Could you check a few things on this model? Use its own coordinates, in mm. Face numbers are marked on the shaded views. A direction names the side the tool comes from. Coordinates: 2 decimals unless noted, no trailing zeros. Order: outer loops, then holes, each group sorted by start corner. A loop starts at its lowest first (then second) coordinate and runs counter-clockwise, first axis right, second up. Notation, with made-up numbers: (20, 70.25) - (29, 70.25) arc R21 cw to (29, 107.25) - close; hole circle Ø10 at (41.5, 88). An arc over 180 degrees is marked (long way). Answer as a JSON object with one key per item and string values. Group by question number.
(1) Imagine slicing it at B-B, the plane z = 39. Write out the boundary of the cut face in (x, y), and give its area (3 significant figures).
(2) We'd pull the mould along X, two halves only. Please class the marked faces 3, 4, 5 and 6: pulls with the +X half, pulls with the -X half, needs draft (parallel to the pull), parting line crosses it, or undercut.
(3) Will these pins go through, and if not, where does the flat tip stop? P1, Ø1, axis at x = -30, y = -20.5, coming from the +Z side; P2, Ø0.6, axis at y = -58, z = 0.5, coming from the +X side; P3, Ø3, axis at y = 42.5, z = 10, coming from the +X side.
(4) Which directions (+Z, -Z, +X, -X, +Y, -Y) give clear straight access to the entire face, cutting with the end or side of a thin tool? Please do the marked faces 1 and 2.
(5) Please list where these lines run through material, in increasing order: probe 1 along X at (y, z) = (32, 39.5); probe 2 along X at (y, z) = (41, 45); probe 3 along Z at (x, y) = (-56, 97).
(6) Imagine slicing it at A-A, the plane x = -19.5. Write out the boundary of the cut face in (y, z).
(7) Imagine slicing it at C-C, the plane y = 83.5. Write out the boundary of the cut face in (x, z), and give its area (3 significant figures).
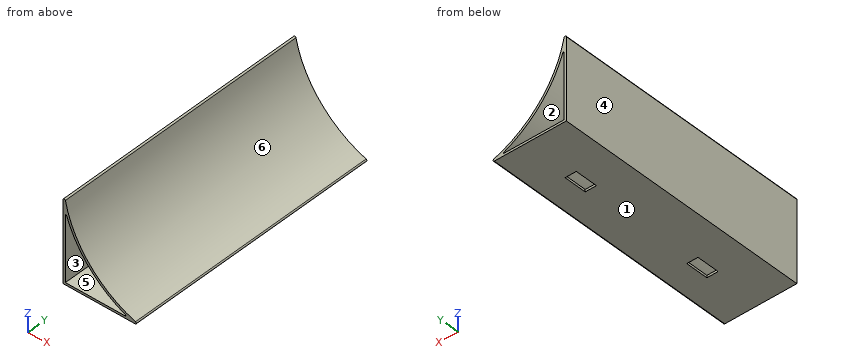
from build123d import *

# Parameters (mm, degrees)
BOSS_EXTRUDE1_DEPTH      = 113.5
BOSS_EXTRUDE1_DEPTH_BACK = 113.5
SKETCH3_W                = 9.8
SKETCH3_H                = 19.8
CUT_EXTRUDE1_DEPTH       = 5


with BuildPart() as part:
    # Sketch2 → Boss-Extrude1 (new, two sides: drawn at the far end of the back side and taken through both)
    with BuildSketch(Plane(origin=(0, 0, 0), x_dir=(-1, 0, 0), z_dir=(0, 1, 0)).offset(-BOSS_EXTRUDE1_DEPTH_BACK)):
        with BuildLine():
            Line((6.944925281, 0), (70, 0))
            Line((70, 0), (70, 70.727517767))
            ThreePointArc((70, 70.727517767), (69.10322059, 71.722176256), (68.02130898, 70.932856238))
            ThreePointArc((68.02130898, 70.932856238), (46.50806151, 28.267371652), (6.627399441, 1.948249619))
            ThreePointArc((6.627399441, 1.948249619), (5.957947667, 0.839142329), (6.944925281, 0))
        make_face()
        with BuildLine():
            Line((68, 58.856286255), (68, 2))
            Line((68, 2), (15.588847456, 2))
            ThreePointArc((15.588847456, 2), (15.099520976, 2.397240103), (15.387714901, 2.957761614))
            ThreePointArc((15.387714901, 2.957761614), (47.071395865, 25.58711402), (67.027291068, 59.019216502))
            ThreePointArc((67.027291068, 59.019216502), (67.582600042, 59.349416291), (68, 58.856286255))
        make_face(mode=Mode.SUBTRACT)
    extrude(amount=BOSS_EXTRUDE1_DEPTH + BOSS_EXTRUDE1_DEPTH_BACK)

    # Sketch3 → Cut-Extrude1 (cut)
    with BuildSketch(Plane(origin=(0, 0, 0), x_dir=(1, 0, 0), z_dir=(0, 0, -1))):
        with Locations((-35, -59.9)):
            Rectangle(SKETCH3_W, SKETCH3_H)
        with Locations((-35, 59.9)):
            Rectangle(SKETCH3_W, SKETCH3_H)
    extrude(amount=-CUT_EXTRUDE1_DEPTH, mode=Mode.SUBTRACT)


solid = part.part
Result set:
{
 "1": {"outline": "(-70, -113.5) - (-68, -113.5) - (-68, 113.5) - (-70, 113.5) - close; (-57.38, -113.5) - (-54.74, -113.5) - (-54.74, 113.5) - (-57.38, 113.5) - close", "area": "1,050 mm^2"},
 "2": {"face 3": "undercut", "face 4": "pulls with the -X half", "face 5": "undercut", "face 6": "pulls with the +X half"},
 "3": {"P1": "stops at z = 14", "P2": "stops at x = -5.97", "P3": "stops at x = -21.64"},
 "4": {"face 1": "-Z, +X, -X, +Y, -Y", "face 2": "+Y, -Y"},
 "5": {"probe 1": "x = -70 to -68, -57.7 to -55.07", "probe 2": "x = -70 to -68, -60.89 to -58.37", "probe 3": "z = 0 to 2, 36.89 to 40.97"},
 "6": {"outline": "(-113.5, 0) - (113.5, 0) - (113.5, 2) - (-113.5, 2) - close; (-113.5, 4.88) - (113.5, 4.88) - (113.5, 7.37) - (-113.5, 7.37) - close"},
 "7": {"outline": "(-70, 0) - (-6.94, 0) arc R1 ccw to (-6.63, 1.95) arc R92.86 cw to (-68.02, 70.93) arc R1 ccw to (-70, 70.73) - close; hole (-68, 2) - (-15.59, 2) arc R0.5 ccw to (-15.39, 2.96) arc R95.07 cw to (-67.03, 59.02) arc R0.5 ccw to (-68, 58.86) - close", "area": "468 mm^2"}
}
